Could you check a few things on this drawing? It's one solid part, dimensions in mm from its lowest x, y, z. A direction names the side the tool comes from. Coordinates: 2 decimals unless noted, no trailing zeros. Order: outer loops, then holes, each group sorted by start corner. A loop starts at its lowest first (then second) coordinate and runs counter-clockwise, first axis right, second up. Notation, with made-up numbers: (13, 53.25) -> (54, 53.25) arc R18 cw to (54, 57.25) -> close; hole circle Ø4 at (-32, -26). An arc over 180 degrees is marked (long way). Use a Markdown table: item, result. Add a question column.
1. For pin 1 Ø2.5 at (x, z) = (1.5, 31.5) entering from -Y; pin 2 Ø3 at (x, z) = (5.5, 26) entering from -Y; pin 3 Ø6 at (x, y) = (9, 3) entering from +Z; pin 4 Ø1.5 at (x, z) = (2, 26) entering from +Y, each with a flat end and sliding along its axis, tell me the tip position at first contact or that it passes through.
2. For the marked faces 1 and 2, which set-ups out of +Z, -Z, +X, -X, +Y, -Y let a thin tool reach every point of the face, with its end or its side?
3. Suppose I cut it at C-C, the plane x = 15. List the corners of the cut face in (y, z) for me, then the cut area to 3 significant figures.
4. Suppose I cut it at A-A, the plane y = 12.5. List the corners of the cut face in (x, z) for me, then the cut area to 3 significant figures.
5. Suppose I cut it at D-D, the plane y = 4.5. List the corners of the cut face in (x, z) for me, then the cut area to 4 significant figures.
6. Suppose I cut it at B-B, the plane x = 9.75. List the corners of the cut face in (y, z) for me.
7. If I drill on line 1 along Y through (x, z) = (15, 1.3); line 2 along Z through (x, y) = (12, 6.75); line 3 along X through (y, z) = (17, 32), over which ranges is the centre line in solid material (lowest first)? Write a range as from..to.
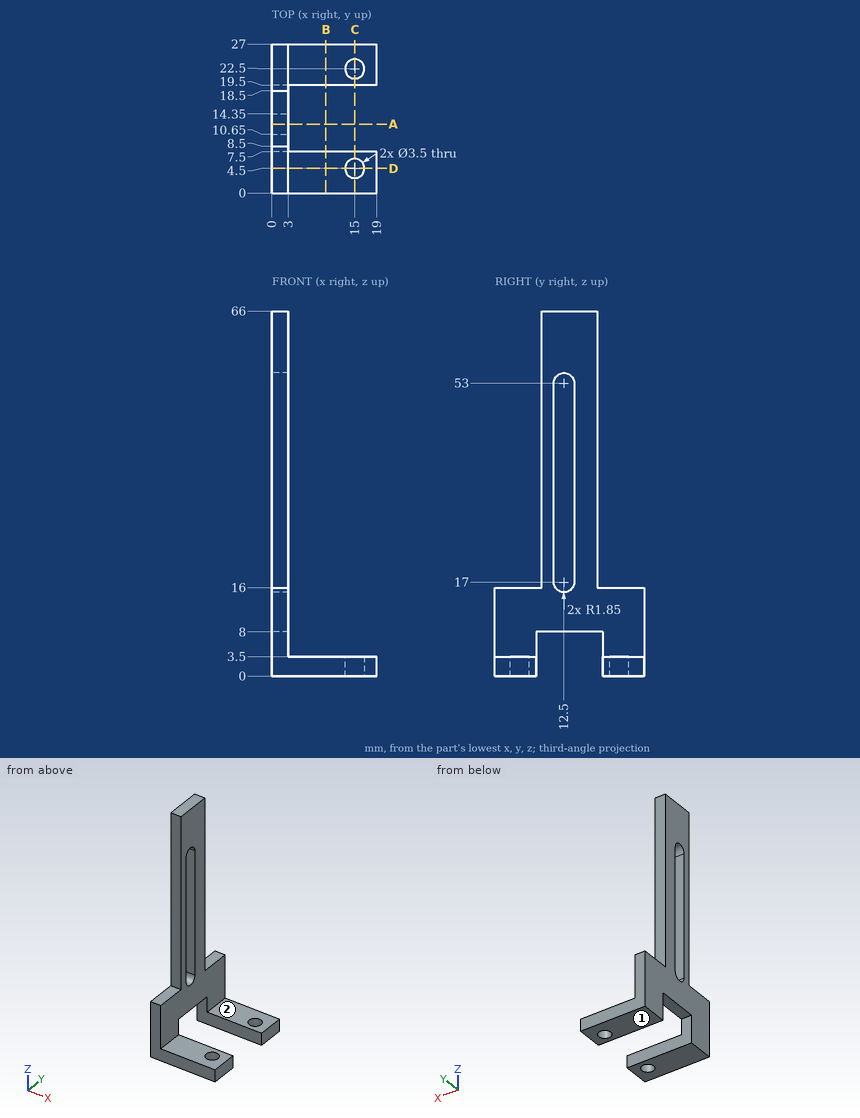
Worked out:
| question | item | result |
|---|---|---|
| 1 | pin 1 | stops at y = 8.5 |
| 1 | pin 2 | passes through |
| 1 | pin 3 | stops at z = 3.5 |
| 1 | pin 4 | stops at y = 18.5 |
| 2 | face 1 | -Z, +X, -X, +Y, -Y |
| 2 | face 2 | +Z, +X, +Y, -Y |
| 3 | outline | (0, 0) -> (2.75, 0) -> (2.75, 3.5) -> (0, 3.5) -> close; (6.25, 0) -> (7.5, 0) -> (7.5, 3.5) -> (6.25, 3.5) -> close; (19.5, 0) -> (20.75, 0) -> (20.75, 3.5) -> (19.5, 3.5) -> close; (24.25, 0) -> (27, 0) -> (27, 3.5) -> (24.25, 3.5) -> close |
| 3 | area | 28.0 mm² |
| 4 | outline | (0, 8) -> (3, 8) -> (3, 15.15) -> (0, 15.15) -> close; (0, 54.85) -> (3, 54.85) -> (3, 66) -> (0, 66) -> close |
| 4 | area | 54.9 mm² |
| 5 | outline | (0, 0) -> (13.25, 0) -> (13.25, 3.5) -> (3, 3.5) -> (3, 16) -> (0, 16) -> close; (16.75, 0) -> (19, 0) -> (19, 3.5) -> (16.75, 3.5) -> close |
| 5 | area | 91.75 mm² |
| 6 | outline | (0, 0) -> (7.5, 0) -> (7.5, 3.5) -> (0, 3.5) -> close; (19.5, 0) -> (27, 0) -> (27, 3.5) -> (19.5, 3.5) -> close |
| 7 | line 1 | y = 0..2.75, 6.25..7.5, 19.5..20.75, 24.25..27 |
| 7 | line 2 | z = 0..3.5 |
| 7 | line 3 | x = 0..3 |
